Build history of the part. All positions in model axes, mm. Give positions to 0.01 mm unless a question says otherwise; leave off trailing zeros. Loops run counter-clockwise (first coordinate to the right, second up) from the corner with the lowest first, then second, coordinate; pieces in that order, holes last.
1) Two-plate mould, pull along X, no slides. Class faces 1 (the cylindrical face through (-49.351, 12.878, 26.215)), 2 (the flat face through (-1, 0, 2)), 3 (the cylindrical face through (-27.84, 12.88, -0.54)), 4 (the cylindrical face through (27.88, 12.88, -0.33)): +X half, -X half, draft (parallel to the pull), parting line (faces both ways), or undercut.
2) Band-saw the part on B-B on z = 0. List the corners of the cut face in (x, y), then the cut area to 3 significant figures.
3) Flat gauge pins, fed straight in: P1, Ø10, axis at x = 34, z = 2, coming from the -Y side; P2, Ø4, axis at x = 25.4, z = 0, coming from the -Y side. Where does each tip first touch, or does it go through?
4) Wall check: line 1 (X direction, y = 14.5, z = 0); line 2 (Z direction, x = -27, y = 11.25); line 3 (Z direction, x = -46, y = 12.25) (3 decimals). Give the ranges that are in metal, low to high.
5) Band-saw the part on A-A on x = 25.4. List the corners of the cut face in (y, z).
```python
from build123d import *

# Parameters (mm, degrees)
SKETCH1_W           = 101.6
SKETCH1_H           = 50.8
BOSS_EXTRUDE1_DEPTH = 25.4
FILLET1_R           = 5.08
FILLET2_R           = 2.54
SKETCH2_R           = 2.5
CUT_EXTRUDE1_DEPTH  = 25.4


with BuildPart() as part:
    # Sketch1 → Boss-Extrude1 (new body)
    with BuildSketch(Plane(origin=(0, 0, 0), x_dir=(1, 0, 0), z_dir=(0, 1, 0))):
        with Locations((0, -2.342718447)):
            Rectangle(SKETCH1_W, SKETCH1_H)
    extrude(amount=BOSS_EXTRUDE1_DEPTH)

    # Fillet1
    fillet1_edges = [part.edges().sort_by_distance(p)[0] for p in [
        (-50.8, 12.7, -23.057281553),
        (-50.8, 12.7, 27.742718447),
    ]]
    fillet(fillet1_edges, radius=FILLET1_R)

    # Fillet2
    fillet2_edges = [part.edges().sort_by_distance(p)[0] for p in [
        (50.8, 12.7, -23.057281553),
        (50.8, 12.7, 27.742718447),
    ]]
    fillet(fillet2_edges, radius=FILLET2_R)

    # Sketch2 → Cut-Extrude1 (cut)
    with BuildSketch(Plane(origin=(0, 25.4, 0), x_dir=(1, 0, 0), z_dir=(0, 1, 0))):
        with Locations(Location((-25.4, 0, 0), (0, 0, 270))):
            Circle(SKETCH2_R)
        with Locations(Location((25.4, 0, 0), (0, 0, 270))):
            Circle(SKETCH2_R)
    extrude(amount=-CUT_EXTRUDE1_DEPTH, mode=Mode.SUBTRACT)


solid = part.part
```
Findings below:
1. face 1: -X half
1. face 2: draft
1. face 3: undercut
1. face 4: undercut
2. outline: (-50.8, 0) - (-27.9, 0) - (-27.9, 25.4) - (-50.8, 25.4) - close; (-22.9, 0) - (22.9, 0) - (22.9, 25.4) - (-22.9, 25.4) - close; (27.9, 0) - (50.8, 0) - (50.8, 25.4) - (27.9, 25.4) - close
2. area: 2,330 mm2
3. P1: stops at y = 0
3. P2: passes through
4. line 1: x = -50.8 to -27.9, -22.9 to 22.9, 27.9 to 50.8
4. line 2: z = -23.06 to -1.92, 1.92 to 27.74
4. line 3: z = -23.05 to 27.735
5. outline: (0, -23.06) - (25.4, -23.06) - (25.4, -2.5) - (0, -2.5) - close; (0, 2.5) - (25.4, 2.5) - (25.4, 27.74) - (0, 27.74) - close
